```python
from build123d import *

# Parameters (mm, degrees)
SKETCH_W        = 557
SKETCH_H        = 770
PAD_DEPTH       = 28
SKETCH001_W     = 220
SKETCH001_H     = 730
SKETCH001_W_2   = 207
POCKET_DEPTH    = 5
SKETCH002_R     = 3
POCKET001_DEPTH = 20


with BuildPart() as part:
    # Sketch → Pad (new body)
    with BuildSketch(Plane.XY):
        with Locations((278.5, 385)):
            Rectangle(SKETCH_W, SKETCH_H)
    extrude(amount=PAD_DEPTH)

    # Sketch001 (on Face6 of Pad) → Pocket (cut)
    with BuildSketch(Plane.XY.offset(28)):
        Polygon((0, 770), (557, 770), (557, 750), (537, 750), (537, 20), (557, 20), (557, 0), (0, 0), (0, 20), (20, 20), (20, 750), (0, 750), align=None)
        with Locations((160, 385)):
            Rectangle(SKETCH001_W, SKETCH001_H, mode=Mode.SUBTRACT)
        with Locations((403.5, 385)):
            Rectangle(SKETCH001_W_2, SKETCH001_H, mode=Mode.SUBTRACT)
    extrude(amount=-POCKET_DEPTH, mode=Mode.SUBTRACT)

    # Sketch002 (on Face6 of Pad) → Pocket001 (cut)
    with BuildSketch(Plane.XY.offset(28)):
        with Locations((100, 40)):
            Circle(SKETCH002_R)
        with Locations((190, 40)):
            Circle(SKETCH002_R)
        with Locations((367, 40)):
            Circle(SKETCH002_R)
        with Locations((457, 40)):
            Circle(SKETCH002_R)
        with Locations((100, 160)):
            Circle(SKETCH002_R)
        with Locations((190, 160)):
            Circle(SKETCH002_R)
        with Locations((367, 160)):
            Circle(SKETCH002_R)
        with Locations((457, 160)):
            Circle(SKETCH002_R)
        with Locations((100, 280)):
            Circle(SKETCH002_R)
        with Locations((190, 280)):
            Circle(SKETCH002_R)
        with Locations((367, 280)):
            Circle(SKETCH002_R)
        with Locations((457, 280)):
            Circle(SKETCH002_R)
        with Locations((100, 400)):
            Circle(SKETCH002_R)
        with Locations((190, 400)):
            Circle(SKETCH002_R)
        with Locations((367, 400)):
            Circle(SKETCH002_R)
        with Locations((457, 400)):
            Circle(SKETCH002_R)
        with Locations((100, 520)):
            Circle(SKETCH002_R)
        with Locations((190, 520)):
            Circle(SKETCH002_R)
        with Locations((367, 520)):
            Circle(SKETCH002_R)
        with Locations((457, 520)):
            Circle(SKETCH002_R)
    extrude(amount=-POCKET001_DEPTH, mode=Mode.SUBTRACT)


with BuildPart() as part_1:
    # Clone placement: moved
    add(part.part.moved(Location((-100, -40, -28))))


solid = part_1.part
```
Geometry: final body of the model. Coordinates: model frame, mm. Coordinates: 2 decimals unless noted, no trailing zeros. Order: outer loops, then holes, each group sorted by start corner. A loop starts at its lowest first (then second) coordinate and runs counter-clockwise, first axis right, second up. Notation, with made-up numbers: (47, -37) -> (89, -37) arc R11 cw to (89, -32) -> close; hole circle Ø1 at (32, 49). An arc over 180 degrees is marked (long way). Write item = value, one per line.
(1) Pull-direction query (X, two-part tool) for faces 1 (the flat face through (457, 340, -14)), 2 (the flat face through (180, 347, -5)), 3 (the flat face through (-100, 340, -14)), 4 (the flat face through (175, -40, -17)); classes: pulls with the +X half, pulls with the -X half, needs draft (parallel to the pull), parting line crosses it, or undercut.
Solved:
face_1 = pulls with the +X half
face_2 = undercut
face_3 = pulls with the -X half
face_4 = needs draft
(2) Line query: line 1 (X direction, y = 240, z = -7.25); line 2 (Y direction, x = 90, z = -12.75); line 3 (X direction, y = 191.5, z = -2.25). Output: solid intervals per line, ascending.
Solved:
line_1 = -100 to -3, 3 to 87, 93 to 264, 270 to 354, 360 to 457
line_2 = -40 to -3, 3 to 117, 123 to 237, 243 to 357, 363 to 477, 483 to 730
line_3 = -100 to -80, -50 to 170, 200 to 407, 437 to 457
(3) Pin query (flat end, axial travel): pin 1 Ø1.8 at (x, y) = (266, 478.5) entering from +Z; pin 2 Ø2.5 at (x, z) = (446.5, -3.5) entering from -Y. Return the tip coordinate at first contact, or that it passes through.
Solved:
pin_1 = -20
pin_2 = -20
(4) Cut plane A-A on y = 332.5. Return loops of the section in (x, z).
Solved:
outline = (-100, -28) -> (457, -28) -> (457, 0) -> (437, 0) -> (437, -5) -> (407, -5) -> (407, 0) -> (200, 0) -> (200, -5) -> (170, -5) -> (170, 0) -> (-50, 0) -> (-50, -5) -> (-80, -5) -> (-80, 0) -> (-100, 0) -> close
